CAD build for the part. Positions are in the model's coordinates, mm. A direction names the side the tool comes from. Give positions to 0.01 mm unless a question says otherwise; leave off trailing zeros. Write each loop counter-clockwise with the first axis right and the second up, starting at its lowest first coordinate (ties: lowest second). Pieces come first, ordered by that corner, then holes. Notation, with made-up numbers: (82, 17.5) - (121, 17.5) arc R16 ccw to (121, 39.5) - close; hole circle Ø10 at (30.25, 45). An arc over 180 degrees is marked (long way). Answer as a JSON object with one key per item and string values.
from build123d import *

# Parameters (mm, degrees)
SKETCH_W        = 30
SKETCH_H        = 30
PAD_DEPTH       = 8
CHAMFER_SIZE    = 2
SKETCH001_W     = 26
SKETCH001_H     = 26
POCKET_DEPTH    = 5
SKETCH002_W     = 24.7
SKETCH002_H     = 12
POCKET001_DEPTH = 5


with BuildPart() as part:
    # Sketch → Pad (new body)
    with BuildSketch(Plane.XY):
        with Locations((15, 15)):
            Rectangle(SKETCH_W, SKETCH_H)
    extrude(amount=PAD_DEPTH)

    # Chamfer
    chamfer_edges = [part.edges().sort_by_distance(p)[0] for p in [
        (15, 0, 8),
        (0, 15, 8),
        (15, 30, 8),
        (30, 15, 8),
    ]]
    chamfer(chamfer_edges, length=CHAMFER_SIZE)

    # Sketch001 (on Face4 of Chamfer) → Pocket (cut)
    with BuildSketch(Plane(origin=(0, 0, 0), x_dir=(1, 0, 0), z_dir=(0, 0, -1))):
        with Locations((15, -15)):
            Rectangle(SKETCH001_W, SKETCH001_H)
    extrude(amount=-POCKET_DEPTH, mode=Mode.SUBTRACT)

    # Sketch002 (on Face8 of Pocket) → Pocket001 (cut)
    with BuildSketch(Plane.XY.offset(8)):
        with Locations((15, 16.17)):
            Rectangle(SKETCH002_W, SKETCH002_H)
    extrude(amount=-POCKET001_DEPTH, mode=Mode.SUBTRACT)


solid = part.part
Item 1: Probe line 1 (X direction, y = 15.5, z = 2.5); line 2 (Y direction, x = 15.5, z = 6). List the from-to ranges inside material, lowest first. Write a range as from..to.
Entries:
{"line 1": "0..2, 28..30", "line 2": "0..10.17, 22.17..30"}
Item 2: Cut at B-B (y = 21.25). Give the cut face in (x, z), and give its area (3 significant figures).
Entries:
{"outline": "(0, 0) - (2, 0) - (2, 5) - (2.65, 5) - (2.65, 8) - (2, 8) - (0, 6) - close; (27.35, 5) - (28, 5) - (28, 0) - (30, 0) - (30, 6) - (28, 8) - (27.35, 8) - close", "area": "31.9 mm2"}
Item 3: Which spindle directions (+Z, -Z, +X, -X, +Y, -Y) get a long thin tool onto all of the face, cutting with end or side? Do faces 1 (the flat face through (15, 28, 2)), 2 (the flat face through (15, 29, 7)), 3 (the flat face through (15, 10.17, 7)). Say none if no direction does.
Entries:
{"face 1": "-Z", "face 2": "+Z, +X, -X, +Y", "face 3": "+Z, -Z"}
Item 4: Flat gauge pins, fed straight in: P1, Ø1, axis at x = 7, y = 8, coming from the -Z side; P2, Ø1, axis at x = 7.5, y = 12.5, coming from the -Z side; P3, Ø0.9, axis at y = 17.5, z = 7, coming from the +X side. Where does each tip first touch, or does it go through?
Entries:
{"P1": "z = 5", "P2": "through", "P3": "x = 29.45"}
Item 5: Cut at C-C (z = 3.5). Give the cut face in (x, y), and give its area (3 significant figures).
Entries:
{"outline": "(0, 0) - (30, 0) - (30, 30) - (0, 30) - close; hole (2, 2) - (28, 2) - (28, 28) - (2, 28) - close", "area": "224 mm2"}
Item 6: Cut at A-A (x = 6). Give the cut face in (y, z).
Entries:
{"outline": "(0, 0) - (2, 0) - (2, 5) - (10.17, 5) - (10.17, 8) - (2, 8) - (0, 6) - close; (22.17, 5) - (28, 5) - (28, 0) - (30, 0) - (30, 6) - (28, 8) - (22.17, 8) - close"}
Item 7: Cut at D-D (y = 24.75). Give the cut face in (x, z).
Entries:
{"outline": "(0, 0) - (2, 0) - (2, 5) - (28, 5) - (28, 0) - (30, 0) - (30, 6) - (28, 8) - (2, 8) - (0, 6) - close"}
Item 8: Mould opens along X. For faces 4 (the flat face through (0, 15, 3)), 5 (the flat face through (15, 9, 5)), 6 (the flat face through (15, 1, 7)), 7 (the flat face through (2.65, 16, 7)) say: +X half, -X half, draft (parallel to the pull), parting line (faces both ways), or undercut.
Entries:
{"face 4": "-X half", "face 5": "undercut", "face 6": "draft", "face 7": "undercut"}
